Design review of the part built by this model. Coordinates are the model's own, in mm. Face numbers are marked on the shaded views. Coordinates: 2 decimals unless noted, no trailing zeros. Write each loop counter-clockwise with the first axis right and the second up, starting at its lowest first coordinate (ties: lowest second). Pieces come first, ordered by that corner, then holes. Notation, with made-up numbers: (-36, -3) - (14, -3) arc R24 ccw to (14, 25) - close; hole circle Ø8 at (87, -13.5). An arc over 180 degrees is marked (long way). Use a Markdown table: item, result.
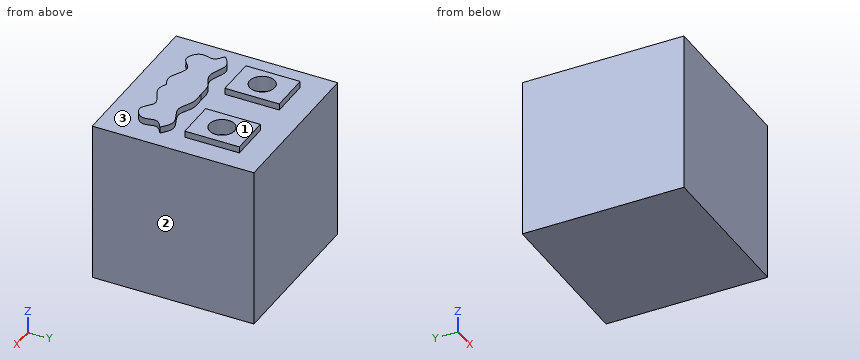
from build123d import *

# Parameters (mm, degrees)
F0_W     = 127
F0_H     = 127
F1_DEPTH = 127
F2_W     = 31.7266828096
F2_H     = 42.8551162527
F3_DEPTH = 5.08
F6_R     = 9.8569317774
F7_DEPTH = 165.1


with BuildPart() as f1:
    # F0 (on Top) → F1 (new body)
    with BuildSketch(Plane.XY):
        with Locations((0.5035735936, -0.4498548806)):
            Rectangle(F0_W, F0_H)
    extrude(amount=F1_DEPTH)

    # F2 (on face) → F3 (join)
    with BuildSketch(Plane.XY.offset(127)):
        Polygon((-45.6073767898, -0.0615948727), (-13.8806939801, -0.1739759996), (-13.8806939801, 42.5792373717), (-45.6073767898, 42.5792373717), align=None)
        with Locations((30.7511825722, 21.1516792453)):
            Rectangle(F2_W, F2_H)
        with BuildLine():
            add(Edge.make_bspline(
                [(50.1263291183, -17.9500691593), (46.7932820736, -15.0577623363), (39.6901265176, -8.8938813577), (24.3847915396, -20.6711745873), (13.3519348493, -10.6155139904), (4.7829499351, -11.2382657266), (0.5035735936, -11.5492697805)],
                knots=[0, 0, 0, 0, 0.2398997898, 0.5112575675, 0.7559205876, 1, 1, 1, 1], degree=3))
            Line((0.5035735936, -11.5492697805), (0.5035735936, -38.543947041))
            add(Edge.make_bspline(
                [(50.1263291183, -17.9500691593), (47.1905685422, -19.9119433554), (41.1553991203, -23.945052613), (48.4880810339, -35.413097395), (33.5272000122, -45.1151840091), (25.8738069034, -29.8543925404), (10.1093672502, -43.4916081263), (3.4299860195, -40.0512557962), (0.5035735936, -38.543947041)],
                knots=[0, 0, 0, 0, 0.1499027043, 0.3081614436, 0.4784483834, 0.6464885348, 0.8451173382, 1, 1, 1, 1], degree=3))
        make_face()
        with BuildLine():
            Line((0.5035735936, -38.543947041), (0.5035735936, -11.5492697805))
            add(Edge.make_bspline(
                [(-49.119181931, -17.9500691593), (-45.7861348863, -15.0577623363), (-38.6829793303, -8.8938813577), (-23.3776443523, -20.6711745873), (-12.344787662, -10.6155139904), (-3.7758027479, -11.2382657266), (0.5035735936, -11.5492697805)],
                knots=[0, 0, 0, 0, 0.2398997898, 0.5112575675, 0.7559205876, 1, 1, 1, 1], degree=3))
            add(Edge.make_bspline(
                [(-49.119181931, -17.9500691593), (-46.1834213549, -19.9119433554), (-40.148251933, -23.945052613), (-47.4809338466, -35.413097395), (-32.5200528249, -45.1151840091), (-24.8666597161, -29.8543925404), (-9.1022200629, -43.4916081263), (-2.4228388322, -40.0512557962), (0.5035735936, -38.543947041)],
                knots=[0, 0, 0, 0, 0.1499027043, 0.3081614436, 0.4784483834, 0.6464885348, 0.8451173382, 1, 1, 1, 1], degree=3))
        make_face()
    extrude(amount=F3_DEPTH)

    # F6 (on offset) → F7 (cut)
    with BuildSketch(Plane.XY.offset(284.48)):
        with Locations((-30.4733738303, 20.5938778818)):
            Circle(F6_R)
        with Locations((30.4733738303, 20.5938778818)):
            Circle(F6_R)
    extrude(amount=-F7_DEPTH, mode=Mode.SUBTRACT)


solid = f1.part
(1) Take a section at B-B on y = 47. Write out the cut boundary in (x, z).
Determined:
| item | result |
|---|---|
| outline | (-63, 0) - (64, 0) - (64, 127) - (-63, 127) - close |
(2) For pin 1 (1.5 mm diameter, centred on x = -32.5, z = 129, fed in from +Y); pin 2 (4 mm diameter, centred on y = 17, z = 130, fed in from +X); pin 3 (12 mm diameter, centred on x = 4.5, y = 39.5, fed in from +Z), all flat-tipped, find the tip position at first contact; note any pin that passes through.
Determined:
| item | result |
|---|---|
| pin 1 | y = 42.58 |
| pin 2 | x = 46.61 |
| pin 3 | z = 127 |
(3) For L1, parallel to Z at x = -12.5, y = 37, list the stretches that pass through material, from the lowest coordinate up. Write a range as from..to.
Determined:
| item | result |
|---|---|
| L1 | 0..127 |
(4) Draft analysis for pull direction X (two halves, no side actions). For the marked faces 1, 2 and 3, state which applies: +X half, -X half, draft (parallel to the pull), parting line (faces both ways), or undercut.
Determined:
| item | result |
|---|---|
| face 1 | draft |
| face 2 | +X half |
| face 3 | undercut |
(5) Take a section at A-A on y = 22.5. Write out the cut boundary in (x, z), and give its area (3 significant figures).
Determined:
| item | result |
|---|---|
| outline | (-63, 0) - (64, 0) - (64, 127) - (46.61, 127) - (46.61, 132.08) - (40.14, 132.08) - (40.14, 119.38) - (20.8, 119.38) - (20.8, 132.08) - (14.89, 132.08) - (14.89, 127) - (-13.88, 127) - (-13.88, 132.08) - (-20.8, 132.08) - (-20.8, 119.38) - (-40.14, 119.38) - (-40.14, 132.08) - (-45.61, 132.08) - (-45.61, 127) - (-63, 127) - close |
| area | 16,000 mm2 |
